from build123d import *

# Parameters (mm, degrees)
F0_R     = 4.0005
F1_DEPTH = 10.16
F0_R_2   = 7.3848382985
F2_DEPTH = 8.1026
F3_SIZE2 = 2.54
F3_SIZE  = 7.62
F5_DEPTH = 25.4
F6_R     = 0.508


with BuildPart() as f1:
    # F0 (on Top) → F1 (new body)
    with BuildSketch(Plane.XY):
        Circle(F0_R)
    extrude(amount=-F1_DEPTH)

    # F0 (on Top) → F2 (join)
    with BuildSketch(Plane.XY):
        Circle(F0_R_2)
        Circle(F0_R, mode=Mode.SUBTRACT)
        Circle(F0_R)
    extrude(amount=F2_DEPTH)

    # F3
    f3_edges = [f1.edges().sort_by_distance(p)[0] for p in [
        (-7.384838, 0, 0),
    ]]
    f3_side = f1.faces().sort_by_distance((-7.384838, 0, 4.0513))[0]
    chamfer(f3_edges, length=F3_SIZE, length2=F3_SIZE2, reference=f3_side)

    # F4 (on face) → F5 (cut)
    with BuildSketch(Plane.XY.offset(8.1026)):
        with BuildLine():
            Line((-6.3938341113, 3.6952296345), (-1.9082015253, 7.1340453905))
            ThreePointArc((-1.9082015253, 7.1340453905), (-4.4930293098, 5.8607614109), (-6.3938341113, 3.6952296345))
        make_face()
        with BuildLine():
            Line((-1.9082015253, 7.1340453905), (3.6952296345, 6.3938341113))
            ThreePointArc((3.6952296345, 6.3938341113), (0.9671326435, 7.3212356296), (-1.9082015253, 7.1340453905))
        make_face()
        with BuildLine():
            Line((3.6952296345, 6.3938341113), (7.1340453905, 1.9082015253))
            ThreePointArc((7.1340453905, 1.9082015253), (5.8607614109, 4.4930293098), (3.6952296345, 6.3938341113))
        make_face()
        with BuildLine():
            Line((7.1340453905, 1.9082015253), (6.3938341113, -3.6952296345))
            ThreePointArc((6.3938341113, -3.6952296345), (7.1327858413, -1.9129042939), (7.3848382985, 0))
            ThreePointArc((7.3848382985, 0), (7.3218716295, 0.9623058433), (7.1340453905, 1.9082015253))
        make_face()
        with BuildLine():
            ThreePointArc((1.9082015253, -7.1340453905), (4.4930293098, -5.8607614109), (6.3938341113, -3.6952296345))
            Line((6.3938341113, -3.6952296345), (1.9082015253, -7.1340453905))
        make_face()
        with BuildLine():
            ThreePointArc((-3.6952296345, -6.3938341113), (-0.9671326435, -7.3212356296), (1.9082015253, -7.1340453905))
            Line((1.9082015253, -7.1340453905), (-3.6952296345, -6.3938341113))
        make_face()
        with BuildLine():
            ThreePointArc((-7.1340453905, -1.9082015253), (-5.8607614109, -4.4930293098), (-3.6952296345, -6.3938341113))
            Line((-3.6952296345, -6.3938341113), (-7.1340453905, -1.9082015253))
        make_face()
        with BuildLine():
            ThreePointArc((-6.3938341113, 3.6952296345), (-7.3212356296, 0.9671326435), (-7.1340453905, -1.9082015253))
            Line((-7.1340453905, -1.9082015253), (-6.3938341113, 3.6952296345))
        make_face()
    extrude(amount=-F5_DEPTH, mode=Mode.SUBTRACT)

    # F6
    f6_edges = [f1.edges().sort_by_distance(p)[0] for p in [
        (-4.0005, 0, -10.16),
    ]]
    fillet(f6_edges, radius=F6_R)


solid = f1.part
Here's how the part is built. I have some questions about the finished solid (model axes, mm). A direction names the side the tool comes from. Coordinates: 2 decimals unless noted, no trailing zeros. Write each loop counter-clockwise with the first axis right and the second up, starting at its lowest first coordinate (ties: lowest second). Pieces come first, ordered by that corner, then holes.
1) If we section it at B-B (x = 0): List the corners of the cut face in (y, z) for me.
Filled in:
outline: (-6.88, 6.11) - (-4.84, 0) - (-4, 0) - (-4, -9.65) arc R0.51 ccw to (-3.49, -10.16) - (3.49, -10.16) arc R0.51 ccw to (4, -9.65) - (4, 0) - (4.84, 0) - (6.88, 6.11) - (6.88, 8.1) - (-6.88, 8.1) - close
2) If we section it at D-D (z = 4): List the corners of the cut face in (x, y) for me.
Filled in:
outline: circle Ø12.36 at (0, 0)
3) Which directions (+Z, -Z, +X, -X, +Y, -Y) give clear straight access to the entire face, cutting with the end or side of a thin tool? Please do faces 1 (the face through (-2, 4, 0)), 2 (the face through (0, 0, 8.103)).
Filled in:
face 1: -Z
face 2: +Z, +X, -X, +Y, -Y
4) If I drill on line 1 (Z direction, x = 2.5, y = 3.75); line 2 (X direction, y = 1, z = 3.75); line 3 (X direction, y = -2.5, z = -8), over which ranges is the centre line in solid material (lowest first)?
Filled in:
line 1: z = 0 to 8.1
line 2: x = -6.01 to 6.01
line 3: x = -3.12 to 3.12
5) If we section it at A-A (z = -4): List the corners of the cut face in (x, y) for me, plus the area to 3 significant figures.
Filled in:
outline: circle Ø8 at (0, 0)
area: 50.3 mm2
6) I'm going to push flat-ended pins straight in: pin 1 (5 mm diameter, centred on x = -0.5, z = -3, fed in from +Y); pin 2 (2 mm diameter, centred on y = -3, z = -6.5, fed in from -X); pin 3 (1.5 mm diameter, centred on y = 4, z = 4, fed in from +X). Where does each tip first touch, or does it pass through?
Filled in:
pin 1: stops at y = 4
pin 2: stops at x = -3.46
pin 3: stops at x = 5.34
